```python
from build123d import *

# Parameters (mm, degrees)
F1_DEPTH      = 30
F2_W          = 30
F2_H          = 2
F3_DEPTH      = 280
F4_W          = 30
F4_H          = 2
F5_DEPTH      = 60
F5_DEPTH_BACK = 2


with BuildPart() as f1:
    # F0 (on Right) → F1 (new body)
    with BuildSketch(Plane.YZ):
        with BuildLine():
            ThreePointArc((-19, 220), (0, 239), (19, 220))
            Line((19, 220), (19, 0))
            Line((19, 0), (21, 0))
            Line((21, 0), (21, 220))
            ThreePointArc((21, 220), (0, 241), (-21, 220))
            Line((-21, 220), (-21, 200))
            Line((-21, 200), (-19, 200))
            Line((-19, 200), (-19, 220))
        make_face()
    extrude(amount=F1_DEPTH)

    # F2 (on face) → F3 (join)
    with BuildSketch(Plane(origin=(0, 21, 0), x_dir=(-1, 0, 0), z_dir=(0, 1, 0))):
        with Locations((-15, 1)):
            Rectangle(F2_W, F2_H)
    extrude(amount=F3_DEPTH)

    # F4 (on face) → F5 (join, two sides)
    with BuildSketch(Plane.XY.offset(2)) as f5_sk:
        with Locations((15, 302)):
            Rectangle(F4_W, F4_H)
    extrude(amount=F5_DEPTH)
    extrude(f5_sk.sketch, amount=-F5_DEPTH_BACK)


solid = f1.part
```
For this review, take the finished solid that the model builds, in its own axes (mm). A direction names the side the tool comes from. Give positions to 0.01 mm unless a question says otherwise; leave off trailing zeros. Loops run counter-clockwise (first coordinate to the right, second up) from the corner with the lowest first, then second, coordinate; pieces in that order, holes last. Notation, with made-up numbers: M 71.5,51 L 126.5,51 A16 cw 126.5,66 Z; hole C 59,22.25 d3. An arc over 180 degrees is marked long. One line per item, written item: value. Start each with the question number.
Q1. Add section A-A (z = 29). Give the boundary of the cut face in (x, y).
Q2. Clearance check with flat-ended pins moving along their axes: pin 1 Ø2 at (x, y) = (19, 302) entering from +Z; pin 2 Ø15 at (x, z) = (14.5, 158.5) entering from +Y; pin 3 Ø6 at (x, z) = (8.5, 153) entering from -Y; pin 4 Ø1 at (x, y) = (6.5, 204.5) entering from -Z. State where each tip first meets the part, or that it passes through.
Q3. For L1, parallel to Y at x = 8, z = 13; L2, parallel to Y at x = 7.25, z = 217; L3, parallel to Y at x = 25.25, z = 156, list the stretches that pass through material, from the lowest coordinate up.
Q4. Add section B-B (x = 11.5). Give the boundary of the cut face in (y, z).
Q5. Add section C-C (y = 0). Give the boundary of the cut face in (x, z).
Q6. Machinability: for faces 5 (the face through (15, 0, 239)), 6 (the face through (15, 301, 32)), which of the approach directions +Z, -Z, +X, -X, +Y, -Y give a long, thin tool a straight path to every point of the face, cutting with its end or side? Answer none if there is none.
Q7. Draft analysis for pull direction Y (two halves, no side actions). For faces 1 (the face through (15, 0, 241)), 2 (the face through (15, -19, 210)), 3 (the face through (15, 21, 109)), 4 (the face through (30, 20, 112)), state which applies: released by +Y, released by -Y, zero draft, split by the parting line, or undercut.
Q8. Add section D-D (z = 80.5). Give the boundary of the cut face in (x, y).
Reply:
1. outline: M 0,19 L 30,19 L 30,21 L 0,21 Z; M 0,301 L 30,301 L 30,303 L 0,303 Z
2. pin 1: z = 62
2. pin 2: y = 21
2. pin 3: y = 19
2. pin 4: z = 0
3. L1: 19 to 21, 301 to 303
3. L2: -21 to -19, 19 to 21
3. L3: 19 to 21
4. outline: M -21,200 L -19,200 L -19,220 A19 cw 19,220 L 19,0 L 303,0 L 303,62 L 301,62 L 301,2 L 21,2 L 21,220 A21 ccw -21,220 Z
5. outline: M 0,239 L 30,239 L 30,241 L 0,241 Z
6. face 5: -Z, +X, -X
6. face 6: +Z, +X, -X
7. face 1: split by the parting line
7. face 2: undercut
7. face 3: undercut
7. face 4: zero draft
8. outline: M 0,19 L 30,19 L 30,21 L 0,21 Z
